Read the model definition and answer for the solid it produces. Units are mm, in the model's axes. Give positions to 0.01 mm unless a question says otherwise; leave off trailing zeros. Order: outer loops, then holes, each group sorted by start corner. A loop starts at its lowest first (then second) coordinate and runs counter-clockwise, first axis right, second up. Notation, with made-up numbers: M 88.5,17.5 L 111.5,17.5 A16 cw 111.5,26.5 Z; hole C 52.25,78.25 d10. An arc over 180 degrees is marked long. One line per item, written item: value. Start each with the question number.
Autodesk Inventor part; units mm, degrees
ref_plane "YZ Plane" through (0, 0, 0) normal (1, 0, 0) x (0, 1, 0)
ref_plane "XZ Plane" through (0, 0, 0) normal (0, 1, 0) x (-1, 0, 0)
ref_plane "XY Plane" through (0, 0, 0) normal (0, 0, 1) x (1, 0, 0)
sketch "Sketch1" plane through (0, 0, 0) normal (0, 0, 1) x (1, 0, 0)
  line L0 (0, 0) -> (-304.8, 0)
  line L1 (-304.8, 0) -> (-304.8, 101.6)
  line L2 (-304.8, 101.6) -> (0, 101.6)
  line L3 (0, 101.6) -> (0, 0)
  circle A0 centre (-292.1, 88.9) radius 3.1
  circle A1 centre (-292.1, 63.5) radius 3.1
  circle A2 centre (-292.1, 38.1) radius 3.1
  circle A3 centre (-292.1, 12.7) radius 3.1
  line L4 (-152.4, 101.6) -> (-152.4, 63.5) construction
  circle A4 centre (-12.7, 88.9) radius 3.1
  circle A5 centre (-12.7, 63.5) radius 3.1
  circle A6 centre (-12.7, 38.1) radius 3.1
  circle A7 centre (-12.7, 12.7) radius 3.1
  dimension "d0" = 304.8
  dimension "d1" = 101.6
  dimension "d2" = 6.2
  dimension "d3" = 12.7
  dimension "d4" = 12.7
  dimension "d7" = 25.4
extrude "Extrusion1" add sketch "Sketch1" along normal blind 6.35
properties part number "shortsides"
Q1. Determine the mould class of faces 1 (the cylindrical face through (-289.236, 39.287, 3.131)), 2 (the flat face through (-155, 52, 6.35)), 3 (the flat face through (-155, 101.6, 3)) for opening direction Y: released by +Y, released by -Y, zero draft, split by the parting line, or undercut.
Q2. This flat-tipped pin is pushed along its axis until it touches: pin 1 (5 mm diameter, centred on x = -292.1, y = 12.7, fed in from +Z). Where does it stop, or does it pass through?
Q3. Find section B-B, the plane x = -292.1. Give the vertices of the cut face in (y, z).
Q4. Find section A-A, the plane y = 12.7. Give the vertices of the cut face in (x, z).
Q5. Consider probe 1 along Y at (x, z) = (-292.1, 4); probe 2 along X at (y, z) = (11.5, 1); probe 3 along X at (y, z) = (11, 3.25). Determine where each line is inside the solid, lowest interval first.
Evaluation:
1. face 1: undercut
1. face 2: zero draft
1. face 3: released by +Y
2. pin 1: through
3. outline: M 0,0 L 9.6,0 L 9.6,6.35 L 0,6.35 Z; M 15.8,0 L 35,0 L 35,6.35 L 15.8,6.35 Z; M 41.2,0 L 60.4,0 L 60.4,6.35 L 41.2,6.35 Z; M 66.6,0 L 85.8,0 L 85.8,6.35 L 66.6,6.35 Z; M 92,0 L 101.6,0 L 101.6,6.35 L 92,6.35 Z
4. outline: M -304.8,0 L -295.2,0 L -295.2,6.35 L -304.8,6.35 Z; M -289,0 L -15.8,0 L -15.8,6.35 L -289,6.35 Z; M -9.6,0 L 0,0 L 0,6.35 L -9.6,6.35 Z
5. probe 1: 0 to 9.6, 15.8 to 35, 41.2 to 60.4, 66.6 to 85.8, 92 to 101.6
5. probe 2: -304.8 to -294.96, -289.24 to -15.56, -9.84 to 0
5. probe 3: -304.8 to -294.69, -289.51 to -15.29, -10.11 to 0
